CAD build for the part. Positions are in the model's coordinates, mm. Give positions to 0.01 mm unless a question says otherwise; leave off trailing zeros. Write each loop counter-clockwise with the first axis right and the second up, starting at its lowest first coordinate (ties: lowest second). Pieces come first, ordered by that corner, then holes. Notation, with made-up numbers: (59, 23) - (110, 23) arc R19 cw to (110, 55) - close; hole circle Ø5 at (-29.75, 13). An arc over 180 degrees is marked (long way). Answer as a JSON object with one key per item and string values.
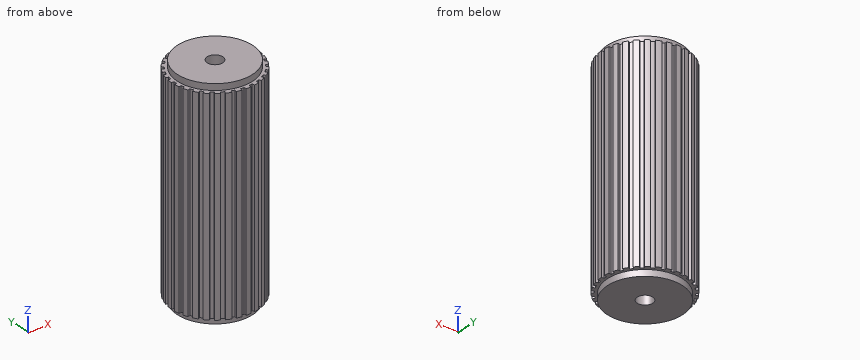
from build123d import *

# Parameters (mm, degrees)
SKETCH1_R           = 60
SKETCH1_R_2         = 12.5
BOSS_EXTRUDE1_DEPTH = 350
SKETCH2_R           = 60
BOSS_EXTRUDE2_DEPTH = 330


with BuildPart() as part:
    # Sketch1 → Boss-Extrude1 (new body)
    with BuildSketch(Plane.XY):
        Circle(SKETCH1_R)
        Circle(SKETCH1_R_2, mode=Mode.SUBTRACT)
    extrude(amount=BOSS_EXTRUDE1_DEPTH)

    # Sketch2 → Boss-Extrude2 (add)
    with BuildSketch(Plane.XY.offset(340)):
        with BuildLine():
            Line((9.367743419, 63.310705124), (10.200923178, 67.230507705))
            ThreePointArc((10.200923178, 67.230507705), (14.137994976, 66.51403685), (18.026103984, 65.567214179))
            Line((18.026103984, 65.567214179), (17.192924224, 61.647411597))
            ThreePointArc((17.192924224, 61.647411597), (19.77708764, 60.867617043), (22.326071498, 59.979550944))
            Line((22.326071498, 59.979550944), (23.956017063, 63.640468622))
            ThreePointArc((23.956017063, 63.640468622), (27.658091729, 62.12109112), (31.264380724, 60.386575478))
            Line((31.264380724, 60.386575478), (29.634435159, 56.725657799))
            ThreePointArc((29.634435159, 56.725657799), (32, 55.425625842), (34.308643121, 54.027002575))
            Line((34.308643121, 54.027002575), (36.664118049, 57.26903568))
            ThreePointArc((36.664118049, 57.26903568), (39.969397156, 55.013155617), (43.136254004, 52.566753661))
            Line((43.136254004, 52.566753661), (40.780779076, 49.324720556))
            ThreePointArc((40.780779076, 49.324720556), (42.824358807, 47.561268831), (44.791762408, 45.713214942))
            Line((44.791762408, 45.713214942), (47.769821142, 48.39467107))
            ThreePointArc((47.769821142, 48.39467107), (50.533848132, 45.500881232), (53.122865993, 42.449512467))
            Line((53.122865993, 42.449512467), (50.144807259, 39.768056338))
            ThreePointArc((50.144807259, 39.768056338), (51.77708764, 37.618256147), (53.317266744, 35.40154046))
            Line((53.317266744, 35.40154046), (56.787753827, 37.405227112))
            ThreePointArc((56.787753827, 37.405227112), (58.889727457, 34), (60.787753827, 30.477023882))
            Line((60.787753827, 30.477023882), (57.317266744, 28.47333723))
            ThreePointArc((57.317266744, 28.47333723), (58.466909289, 26.031145157), (59.512550678, 23.542648785))
            Line((59.512550678, 23.542648785), (63.323789171, 24.780995239))
            ThreePointArc((63.323789171, 24.780995239), (64.671843108, 21.013155617), (65.795925126, 17.172543108))
            Line((65.795925126, 17.172543108), (61.984686633, 15.934196655))
            ThreePointArc((61.984686633, 15.934196655), (62.601446447, 13.306348212), (63.106850574, 10.654830388))
            Line((63.106850574, 10.654830388), (67.092271067, 11.073714961))
            ThreePointArc((67.092271067, 11.073714961), (67.627488885, 7.107935502), (67.928498773, 3.117539798))
            Line((67.928498773, 3.117539798), (63.94307828, 2.698655225))
            ThreePointArc((63.94307828, 2.698655225), (64, 0), (63.94307828, -2.698655225))
            Line((63.94307828, -2.698655225), (67.928498773, -3.117539798))
            ThreePointArc((67.928498773, -3.117539798), (67.627488885, -7.107935502), (67.092271067, -11.073714961))
            Line((67.092271067, -11.073714961), (63.106850574, -10.654830388))
            ThreePointArc((63.106850574, -10.654830388), (62.601446447, -13.306348212), (61.984686633, -15.934196655))
            Line((61.984686633, -15.934196655), (65.795925126, -17.172543108))
            ThreePointArc((65.795925126, -17.172543108), (64.671843108, -21.013155617), (63.323789171, -24.780995239))
            Line((63.323789171, -24.780995239), (59.512550678, -23.542648785))
            ThreePointArc((59.512550678, -23.542648785), (58.466909289, -26.031145157), (57.317266744, -28.47333723))
            Line((57.317266744, -28.47333723), (60.787753827, -30.477023882))
            ThreePointArc((60.787753827, -30.477023882), (58.889727457, -34), (56.787753827, -37.405227112))
            Line((56.787753827, -37.405227112), (53.317266744, -35.40154046))
            ThreePointArc((53.317266744, -35.40154046), (51.77708764, -37.618256147), (50.144807259, -39.768056338))
            Line((50.144807259, -39.768056338), (53.122865993, -42.449512467))
            ThreePointArc((53.122865993, -42.449512467), (50.533848132, -45.500881232), (47.769821142, -48.39467107))
            Line((47.769821142, -48.39467107), (44.791762408, -45.713214942))
            ThreePointArc((44.791762408, -45.713214942), (42.824358807, -47.561268831), (40.780779076, -49.324720556))
            Line((40.780779076, -49.324720556), (43.136254004, -52.566753661))
            ThreePointArc((43.136254004, -52.566753661), (39.969397156, -55.013155617), (36.664118049, -57.26903568))
            Line((36.664118049, -57.26903568), (34.308643121, -54.027002575))
            ThreePointArc((34.308643121, -54.027002575), (32, -55.425625842), (29.634435159, -56.725657799))
            Line((29.634435159, -56.725657799), (31.264380724, -60.386575478))
            ThreePointArc((31.264380724, -60.386575478), (27.658091729, -62.12109112), (23.956017063, -63.640468622))
            Line((23.956017063, -63.640468622), (22.326071498, -59.979550944))
            ThreePointArc((22.326071498, -59.979550944), (19.77708764, -60.867617043), (17.192924224, -61.647411597))
            Line((17.192924224, -61.647411597), (18.026103984, -65.567214179))
            ThreePointArc((18.026103984, -65.567214179), (14.137994976, -66.51403685), (10.200923178, -67.230507705))
            Line((10.200923178, -67.230507705), (9.367743419, -63.310705124))
            ThreePointArc((9.367743419, -63.310705124), (6.689821649, -63.649401304), (4, -63.874877691))
            Line((4, -63.874877691), (4, -67.882250994))
            ThreePointArc((4, -67.882250994), (0, -68), (-4, -67.882250994))
            Line((-4, -67.882250994), (-4, -63.874877691))
            ThreePointArc((-4, -63.874877691), (-6.689821649, -63.649401304), (-9.367743419, -63.310705124))
            Line((-9.367743419, -63.310705124), (-10.200923178, -67.230507705))
            ThreePointArc((-10.200923178, -67.230507705), (-14.137994976, -66.51403685), (-18.026103984, -65.567214179))
            Line((-18.026103984, -65.567214179), (-17.192924224, -61.647411597))
            ThreePointArc((-17.192924224, -61.647411597), (-19.77708764, -60.867617043), (-22.326071498, -59.979550944))
            Line((-22.326071498, -59.979550944), (-23.956017063, -63.640468622))
            ThreePointArc((-23.956017063, -63.640468622), (-27.658091729, -62.12109112), (-31.264380724, -60.386575478))
            Line((-31.264380724, -60.386575478), (-29.634435159, -56.725657799))
            ThreePointArc((-29.634435159, -56.725657799), (-32, -55.425625842), (-34.308643121, -54.027002575))
            Line((-34.308643121, -54.027002575), (-36.664118049, -57.26903568))
            ThreePointArc((-36.664118049, -57.26903568), (-39.969397156, -55.013155617), (-43.136254004, -52.566753661))
            Line((-43.136254004, -52.566753661), (-40.780779076, -49.324720556))
            ThreePointArc((-40.780779076, -49.324720556), (-42.824358807, -47.561268831), (-44.791762408, -45.713214942))
            Line((-44.791762408, -45.713214942), (-47.769821142, -48.39467107))
            ThreePointArc((-47.769821142, -48.39467107), (-50.533848132, -45.500881232), (-53.122865993, -42.449512467))
            Line((-53.122865993, -42.449512467), (-50.144807259, -39.768056338))
            ThreePointArc((-50.144807259, -39.768056338), (-51.77708764, -37.618256147), (-53.317266744, -35.40154046))
            Line((-53.317266744, -35.40154046), (-56.787753827, -37.405227112))
            ThreePointArc((-56.787753827, -37.405227112), (-58.889727457, -34), (-60.787753827, -30.477023882))
            Line((-60.787753827, -30.477023882), (-57.317266744, -28.47333723))
            ThreePointArc((-57.317266744, -28.47333723), (-58.466909289, -26.031145157), (-59.512550678, -23.542648785))
            Line((-59.512550678, -23.542648785), (-63.323789171, -24.780995239))
            ThreePointArc((-63.323789171, -24.780995239), (-64.671843108, -21.013155617), (-65.795925126, -17.172543108))
            Line((-65.795925126, -17.172543108), (-61.984686633, -15.934196655))
            ThreePointArc((-61.984686633, -15.934196655), (-62.601446447, -13.306348212), (-63.106850574, -10.654830388))
            Line((-63.106850574, -10.654830388), (-67.092271067, -11.073714961))
            ThreePointArc((-67.092271067, -11.073714961), (-67.627488885, -7.107935502), (-67.928498773, -3.117539798))
            Line((-67.928498773, -3.117539798), (-63.94307828, -2.698655225))
            ThreePointArc((-63.94307828, -2.698655225), (-64, 0), (-63.94307828, 2.698655225))
            Line((-63.94307828, 2.698655225), (-67.928498773, 3.117539798))
            ThreePointArc((-67.928498773, 3.117539798), (-67.627488885, 7.107935502), (-67.092271067, 11.073714961))
            Line((-67.092271067, 11.073714961), (-63.106850574, 10.654830388))
            ThreePointArc((-63.106850574, 10.654830388), (-62.601446447, 13.306348212), (-61.984686633, 15.934196655))
            Line((-61.984686633, 15.934196655), (-65.795925126, 17.172543108))
            ThreePointArc((-65.795925126, 17.172543108), (-64.671843108, 21.013155617), (-63.323789171, 24.780995239))
            Line((-63.323789171, 24.780995239), (-59.512550678, 23.542648785))
            ThreePointArc((-59.512550678, 23.542648785), (-58.466909289, 26.031145157), (-57.317266744, 28.47333723))
            Line((-57.317266744, 28.47333723), (-60.787753827, 30.477023882))
            ThreePointArc((-60.787753827, 30.477023882), (-58.889727457, 34), (-56.787753827, 37.405227112))
            Line((-56.787753827, 37.405227112), (-53.317266744, 35.40154046))
            ThreePointArc((-53.317266744, 35.40154046), (-51.77708764, 37.618256147), (-50.144807259, 39.768056338))
            Line((-50.144807259, 39.768056338), (-53.122865993, 42.449512467))
            ThreePointArc((-53.122865993, 42.449512467), (-50.533848132, 45.500881232), (-47.769821142, 48.39467107))
            Line((-47.769821142, 48.39467107), (-44.791762408, 45.713214942))
            ThreePointArc((-44.791762408, 45.713214942), (-42.824358807, 47.561268831), (-40.780779076, 49.324720556))
            Line((-40.780779076, 49.324720556), (-43.136254004, 52.566753661))
            ThreePointArc((-43.136254004, 52.566753661), (-39.969397156, 55.013155617), (-36.664118049, 57.26903568))
            Line((-36.664118049, 57.26903568), (-34.308643121, 54.027002575))
            ThreePointArc((-34.308643121, 54.027002575), (-32, 55.425625842), (-29.634435159, 56.725657799))
            Line((-29.634435159, 56.725657799), (-31.264380724, 60.386575478))
            ThreePointArc((-31.264380724, 60.386575478), (-27.658091729, 62.12109112), (-23.956017063, 63.640468622))
            Line((-23.956017063, 63.640468622), (-22.326071498, 59.979550944))
            ThreePointArc((-22.326071498, 59.979550944), (-19.77708764, 60.867617043), (-17.192924224, 61.647411597))
            Line((-17.192924224, 61.647411597), (-18.026103984, 65.567214179))
            ThreePointArc((-18.026103984, 65.567214179), (-14.137994976, 66.51403685), (-10.200923178, 67.230507705))
            Line((-10.200923178, 67.230507705), (-9.367743419, 63.310705124))
            ThreePointArc((-9.367743419, 63.310705124), (-6.689821649, 63.649401304), (-4, 63.874877691))
            Line((-4, 63.874877691), (-4, 67.882250994))
            ThreePointArc((-4, 67.882250994), (0, 68), (4, 67.882250994))
            Line((4, 67.882250994), (4, 63.874877691))
            ThreePointArc((4, 63.874877691), (6.689821649, 63.649401304), (9.367743419, 63.310705124))
        make_face()
        Circle(SKETCH2_R, mode=Mode.SUBTRACT)
    extrude(amount=-BOSS_EXTRUDE2_DEPTH)


solid = part.part
Item 1: Cut at A-A (x = 0). Give the cut face in (y, z).
Entries:
{"outline": "(-68, 10) - (-60, 10) - (-60, 0) - (-12.5, 0) - (-12.5, 350) - (-60, 350) - (-60, 340) - (-68, 340) - close; (12.5, 0) - (60, 0) - (60, 10) - (68, 10) - (68, 340) - (60, 340) - (60, 350) - (12.5, 350) - close"}
Item 2: Flat gauge pins, fed straight in: P1, Ø8, axis at x = -53, y = 6.5, coming from the -Z side; P2, Ø2, axis at y = -66.5, z = 142.5, coming from the +X side; P3, Ø2, axis at y = 65, z = 107, coming from the -X side; P4, Ø6, axis at x = 45, z = 114, coming from the -Y side. Where does each tip first touch, or does it go through?
Entries:
{"P1": "z = 0", "P2": "x = 18.03", "P3": "x = -18.03", "P4": "y = -53.48"}
Item 3: Probe line 1 (Y direction, x = -1, z = 327.5); line 2 (Y direction, x = -25, z = 245); line 3 (X direction, y = 10, z = 305). List the from-to ranges inside material, lowest first. Write a range as from..to.
Entries:
{"line 1": "-67.99..-12.46, 12.46..67.99", "line 2": "-63.24..63.24", "line 3": "-67.26..-7.5, 7.5..67.26"}
